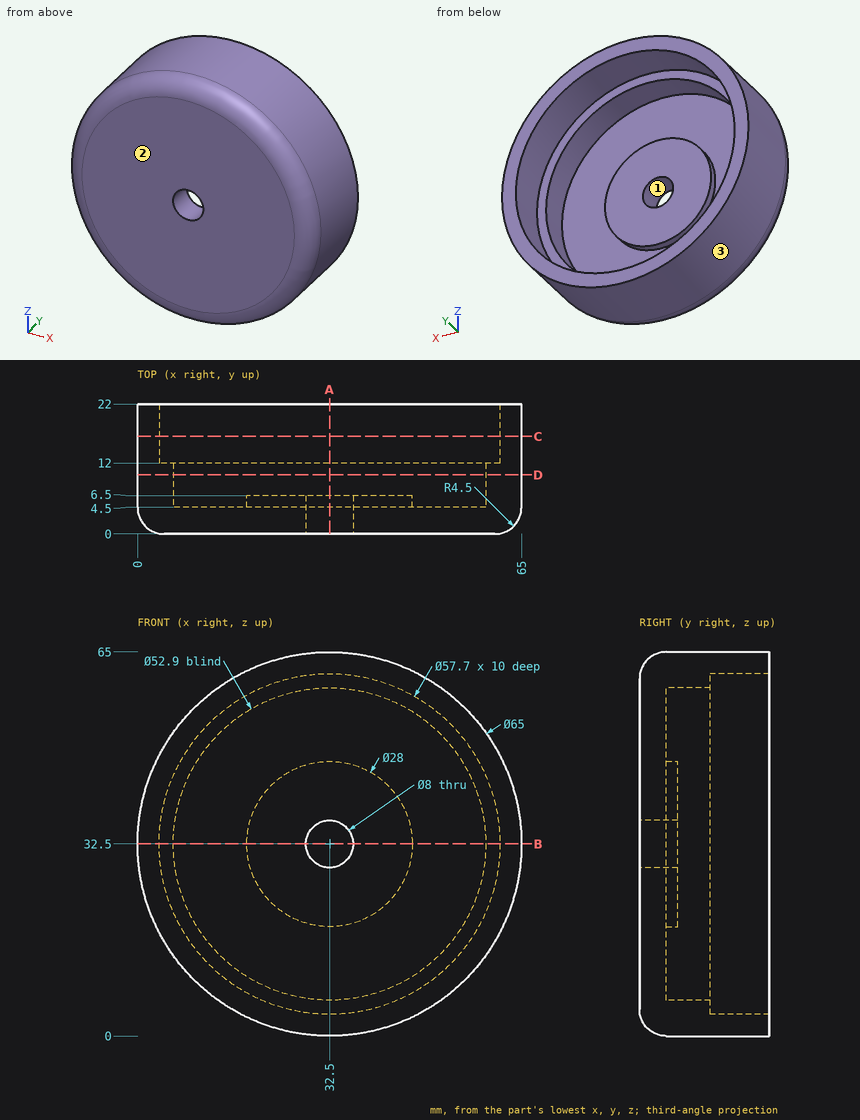
Source: three-view drawing plus pictorial views. Frame: mm from the lowest corner of the part. Round coordinates to 2 decimals unless told otherwise and drop trailing zeros. Order: outer loops, then holes, each group sorted by start corner. A loop starts at its lowest first (then second) coordinate and runs counter-clockwise, first axis right, second up. Notation, with made-up numbers: (47.25, 60.5) -> (89.25, 60.5) arc R33 ccw to (89.25, 98.5) -> close; hole circle Ø3 at (31.5, -34.5). An arc over 180 degrees is marked (long way). Use CSV: the item, a comma, the result in double quotes. Start each with the question number.
1) Section C-C (y = 16.5). Return the cut outline in (x, z), and give its area (3 significant figures).
2) First-contact query: pin 1 Ø4 at (x, y) = (17, 12) entering from +Z; pin 2 Ø6.5 at (x, z) = (32.5, 32.5) entering from +Y; pin 3 Ø6 at (y, z) = (11.5, 18) entering from +X; pin 4 Ø1.5 at (x, y) = (44.5, 6) entering from -Z. Flat tips, straight axial feed; report the tip coordinate or a pass-through.
3) Section B-B (z = 32.5). Return the cut outline in (x, y), and give its area (3 significant figures).
4) Material intervals for line 1 along X through (y, z) = (17, 32.5); line 2 along X through (y, z) = (8.5, 32.5), sorted ascending. Write a range as from..to.
5) Draft query along Z for the marked faces 1, 2 and 3. Return one class per face: +Z half, -Z half, draft (parallel to the pull), parting line (faces both ways), or undercut.
6) Section A-A (x = 32.5). Return the cut outline in (y, z).
7) Section D-D (y = 10). Return the cut outline in (x, z).
Returned:
1,outline,"circle Ø65 at (32.5, 32.5); hole circle Ø57.7 at (32.5, 32.5)"
1,area,"703 mm²"
2,pin 1,"stops at z = 62.06"
2,pin 2,"passes through"
2,pin 3,"stops at x = 62.9"
2,pin 4,"stops at z = 2.01"
3,outline,"(0, 4.5) arc R4.5 ccw to (4.5, 0) -> (28.5, 0) -> (28.5, 6.5) -> (18.5, 6.5) -> (18.5, 4.5) -> (6.05, 4.5) -> (6.05, 12) -> (3.65, 12) -> (3.65, 22) -> (0, 22) -> close; (36.5, 0) -> (60.5, 0) arc R4.5 ccw to (65, 4.5) -> (65, 22) -> (61.35, 22) -> (61.35, 12) -> (58.95, 12) -> (58.95, 4.5) -> (46.5, 4.5) -> (46.5, 6.5) -> (36.5, 6.5) -> close"
3,area,"452 mm²"
4,line 1,"x = 0..3.65, 61.35..65"
4,line 2,"x = 0..6.05, 58.95..65"
5,face 1,"undercut"
5,face 2,"draft"
5,face 3,"parting line"
6,outline,"(0, 4.5) arc R4.5 ccw to (4.5, 0) -> (22, 0) -> (22, 3.65) -> (12, 3.65) -> (12, 6.05) -> (4.5, 6.05) -> (4.5, 18.5) -> (6.5, 18.5) -> (6.5, 28.5) -> (0, 28.5) -> close; (0, 36.5) -> (6.5, 36.5) -> (6.5, 46.5) -> (4.5, 46.5) -> (4.5, 58.95) -> (12, 58.95) -> (12, 61.35) -> (22, 61.35) -> (22, 65) -> (4.5, 65) arc R4.5 ccw to (0, 60.5) -> close"
7,outline,"circle Ø65 at (32.5, 32.5); hole circle Ø52.9 at (32.5, 32.5)"
